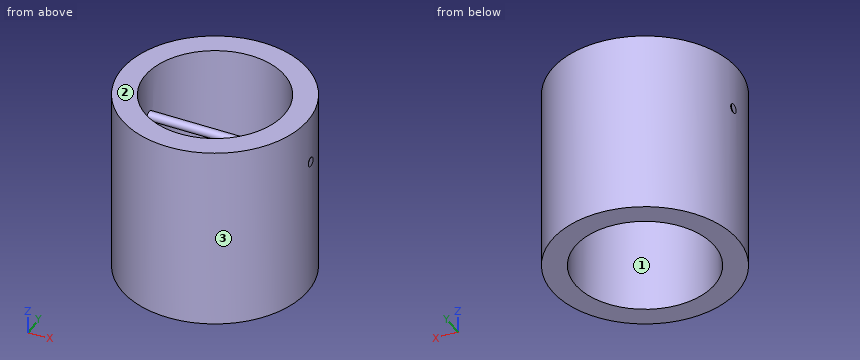
from build123d import *

# Parameters (mm, degrees)
BOSS_EXTRUDE1_DEPTH      = 20
BOSS_EXTRUDE1_DEPTH_BACK = 20
SKETCH1_R                = 20
SKETCH1_R_2              = 15
BOSS_EXTRUDE2_START      = -20
SKETCH2_R                = 1
BOSS_EXTRUDE2_DEPTH      = 40


with BuildPart() as part:
    # Sketch1 → Boss-Extrude1 (new, two sides: drawn at the far end of the back side and taken through both)
    with BuildSketch(Plane.XY.offset(-BOSS_EXTRUDE1_DEPTH_BACK)):
        Circle(SKETCH1_R)
        Circle(SKETCH1_R_2, mode=Mode.SUBTRACT)
    extrude(amount=BOSS_EXTRUDE1_DEPTH + BOSS_EXTRUDE1_DEPTH_BACK)

    # Sketch2 → Boss-Extrude2 (add)
    with BuildSketch(Plane(origin=(0, 0, 0), x_dir=(0, 0, -1), z_dir=(1, 0, 0)).offset(BOSS_EXTRUDE2_START)):
        with Locations(Location((-9.558885453, 1.461191935, 0), (0, 0, 180))):
            Circle(SKETCH2_R)
    extrude(amount=BOSS_EXTRUDE2_DEPTH)


solid = part.part
Can you work these out from the model? Positions are in its coordinate system, mm. Face numbers are marked on the shaded views. Round coordinates to 2 decimals unless told otherwise and drop trailing zeros. Write each loop counter-clockwise with the first axis right and the second up, starting at its lowest first coordinate (ties: lowest second). Pieces come first, ordered by that corner, then holes. Notation, with made-up numbers: (29.25, -13) -> (46.25, -13) arc R33 ccw to (46.25, 15) -> close; hole circle Ø8 at (67.5, 75). An arc over 180 degrees is marked (long way). One line per question, with ' | ' between items. Start each with the question number.
1) Suppose I cut it at C-C on z = 5.5. Write out the boundary of the cut face in (x, y), then the cut area to 3 significant figures.
2) Suppose I cut it at A-A on x = 0. Write out the boundary of the cut face in (y, z).
3) Suppose I cut it at D-D on x = 14. Write out the boundary of the cut face in (y, z).
4) I'm going to push flat-ended pins straight in: P1, Ø2, axis at y = -16, z = 7, coming from the -X side; P2, Ø12, axis at x = -4, z = -9.5, coming from the +Y side; P3, Ø1.5, axis at y = 5.5, z = -13, coming from the +X side; P4, Ø8, axis at y = -1, z = -3.5, coming from the -X side. Where does each tip first touch, or does it pass through?
5) I need wall thicknesses on line 1 (Y direction, x = 0, z = 3); line 2 (X direction, y = -0.5, z = 9); line 3 (Y direction, x = -2, z = 9.5). Which ranges of each line are inside material? Lowest first, please. Write a range as [from, to].
6) Suppose I cut it at B-B on y = -12.5. Write out the boundary of the cut face in (x, z).
7) If we mould it in two halves opening along X, with no side actions, what happens to the marked faces 1, 2 and 3? For each: released by +X, released by -X, zero draft, split by the parting line, or undercut.
Return value:
1) outline: circle Ø40 at (0, 0); hole circle Ø30 at (0, 0) | area: 550 mm2
2) outline: (-20, -20) -> (-15, -20) -> (-15, 20) -> (-20, 20) -> close; circle Ø2 at (1.46, 9.56); (15, -20) -> (20, -20) -> (20, 20) -> (15, 20) -> close
3) outline: (-14.28, -20) -> (-5.39, -20) -> (-5.39, 20) -> (-14.28, 20) -> close; circle Ø2 at (1.46, 9.56); (5.39, -20) -> (14.28, -20) -> (14.28, 20) -> (5.39, 20) -> close
4) P1: stops at x = -13.23 | P2: stops at y = 20 | P3: stops at x = 19.43 | P4: stops at x = -20
5) line 1: y = [-20, -15], [15, 20] | line 2: x = [-19.99, -14.99], [14.99, 19.99] | line 3: y = [-19.9, -14.87], [0.46, 2.46], [14.87, 19.9]
6) outline: (-15.61, -20) -> (-8.29, -20) -> (-8.29, 20) -> (-15.61, 20) -> close; (8.29, -20) -> (15.61, -20) -> (15.61, 20) -> (8.29, 20) -> close
7) face 1: undercut | face 2: zero draft | face 3: split by the parting line
